Geometry: final body of the model. Coordinates: model frame, mm. Face numbers are marked on the shaded views. A direction names the side the tool comes from. Round coordinates to 2 decimals unless told otherwise and drop trailing zeros. Order: outer loops, then holes, each group sorted by start corner. A loop starts at its lowest first (then second) coordinate and runs counter-clockwise, first axis right, second up. Notation, with made-up numbers: M 40,-23.75 L 73,-23.75 A9 ccw 73,-8.75 Z; hole C 0,80.25 d1. An arc over 180 degrees is marked long. Put each result on its own line as item: value. Start each with the question number.
1) Section C-C, the plane y = 7.5. Return loops of the section in (x, z), then the cut area to 3 significant figures.
2) Material intervals for probe 1 along Z at (x, y) = (8, 55.5); probe 2 along Z at (x, y) = (10.5, 35.5); probe 3 along X at (y, z) = (16.5, -6), sorted ascending. Write a range as [from, to].
3) Access query for the marked faces 4, 5 and 6. Directions: +Z, -Z, +X, -X, +Y, -Y. A direction counts if a zero-diameter tool reaches every point of the face in a straight line with its end or side. Return the directions, or none.
4) Draft query along Z for the marked faces 1, 2 and 3. Return one class per face: pulls with the +Z half, pulls with the -Z half, needs draft (parallel to the pull), parting line crosses it, or undercut.
5) Section B-B, the plane z = -8. Return loops of the section in (x, y), then the cut area to 3 significant figures.
6) First-contact query: P1, Ø11.5, axis at x = 11, y = 23.5, coming from the -Z side; P2, Ø5, axis at x = 11, z = -3.5, coming from the -Y side; P3, Ø3, axis at x = 14.5, z = -18.5, coming from the -Y side. Flat tips, straight axial feed; report the tip coordinate or a pass-through.
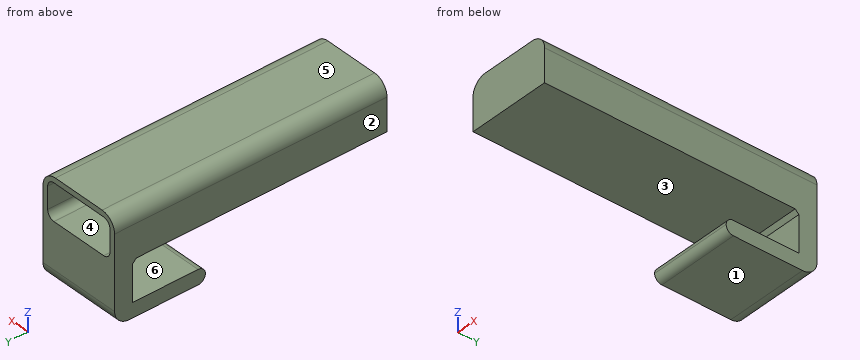
from build123d import *

# Parameters (mm, degrees)
BOSS_EXTRUDE1_DEPTH = 23
SKETCH3_W           = 20
SKETCH3_H           = 10
CUT_EXTRUDE1_DEPTH  = 73
CHAMFER1_SIZE       = 1
FILLET1_R           = 4
FILLET2_R           = 2
FILLET3_R           = 4
FILLET4_R           = 2


with BuildPart() as part:
    # Sketch2 → Boss-Extrude1 (new body)
    with BuildSketch(Plane(origin=(0, 0, 0), x_dir=(0, 0, -1), z_dir=(1, 0, 0))):
        Polygon((0, 0), (13, 0), (13, 70), (24, 70), (24, 50), (28, 50), (28, 75), (0, 75), align=None)
    extrude(amount=BOSS_EXTRUDE1_DEPTH)

    # Sketch3 → Cut-Extrude1 (cut)
    with BuildSketch(Plane(origin=(0, 75, 0), x_dir=(1, 0, 0), z_dir=(0, 1, 0))):
        with Locations((11.5, 6.5)):
            Rectangle(SKETCH3_W, SKETCH3_H)
    extrude(amount=-CUT_EXTRUDE1_DEPTH, mode=Mode.SUBTRACT)

    # Chamfer1
    chamfer1_edges = [part.edges().sort_by_distance(p)[0] for p in [
        (11.5, 70, -13),
    ]]
    chamfer(chamfer1_edges, length=CHAMFER1_SIZE)

    # Fillet1
    fillet1_edges = [part.edges().sort_by_distance(p)[0] for p in [
        (0, 37.5, 0),
        (23, 37.5, 0),
    ]]
    fillet(fillet1_edges, radius=FILLET1_R)

    # Fillet2
    fillet2_edges = [part.edges().sort_by_distance(p)[0] for p in [
        (1.5, 38.5, -11.5),
        (21.5, 38.5, -11.5),
        (21.5, 38.5, -1.5),
        (1.5, 38.5, -1.5),
    ]]
    fillet(fillet2_edges, radius=FILLET2_R)

    # Fillet3
    fillet3_edges = [part.edges().sort_by_distance(p)[0] for p in [
        (11.5, 75, -28),
    ]]
    fillet(fillet3_edges, radius=FILLET3_R)

    # Fillet4
    fillet4_edges = [part.edges().sort_by_distance(p)[0] for p in [
        (11.5, 50, -28),
        (11.5, 50, -24),
    ]]
    fillet(fillet4_edges, radius=FILLET4_R - 0.0001)  # a hair under: the kernel refuses the full size


solid = part.part
Result sheet:
1. outline: M 0,-13 L 23,-13 L 23,-4 A4 ccw 19,0 L 4,0 A4 ccw 0,-4 Z; hole M 1.5,-9.5 A2 ccw 3.5,-11.5 L 19.5,-11.5 A2 ccw 21.5,-9.5 L 21.5,-3.5 A2 ccw 19.5,-1.5 L 3.5,-1.5 A2 ccw 1.5,-3.5 Z
1. area: 95.6 mm2
2. probe 1: z = [-28, -24], [-13, -11.5], [-1.5, 0]
2. probe 2: z = [-13, -11.5], [-1.5, 0]
2. probe 3: x = [0, 1.5], [21.5, 23]
3. face 4: +Y
3. face 5: +Z, +X, -X, +Y, -Y
3. face 6: +X, -X, -Y
4. face 1: pulls with the -Z half
4. face 2: needs draft
4. face 3: undercut
5. outline: M 0,0 L 23,0 L 23,75 L 21.5,75 L 21.5,2 L 1.5,2 L 1.5,75 L 0,75 Z
5. area: 265 mm2
6. P1: stops at z = -13
6. P2: stops at y = 0
6. P3: stops at y = 70
